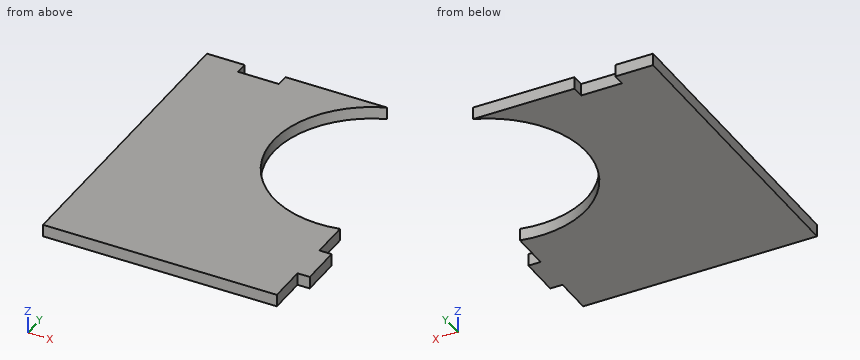
from build123d import *

# Parameters (mm, degrees)
SALIENTE_EXTRUIR1_DEPTH = 3


with BuildPart() as part:
    # Croquis1 → Saliente-Extruir1 (new body)
    with BuildSketch(Plane.XY):
        with BuildLine():
            Line((-3, 0.83840696), (-60.3, 0.83840696))
            Line((-60.3, 0.83840696), (-60.3, 75.83840696))
            Line((-60.3, 75.83840696), (-51.05, 75.83840696))
            Line((-51.05, 75.83840696), (-51.05, 72.83840696))
            Line((-51.05, 72.83840696), (-41.05, 72.83840696))
            Line((-41.05, 72.83840696), (-41.05, 75.83840696))
            Line((-41.05, 75.83840696), (-16.187910348, 75.83840696))
            ThreePointArc((-16.187910348, 75.83840696), (-30.919705343, 46.687711053), (-3, 29.73840696))
            Line((-3, 29.73840696), (-3, 20.28840696))
            Line((-3, 20.28840696), (0, 20.28840696))
            Line((0, 20.28840696), (0, 10.28840696))
            Line((0, 10.28840696), (-3, 10.28840696))
            Line((-3, 10.28840696), (-3, 0.83840696))
        make_face()
    extrude(amount=SALIENTE_EXTRUIR1_DEPTH)


solid = part.part
CAD build for the part. Positions are in the model's coordinates, mm. Give positions to 0.01 mm unless a question says otherwise; leave off trailing zeros. Loops run counter-clockwise (first coordinate to the right, second up) from the corner with the lowest first, then second, coordinate; pieces in that order, holes last. Notation, with made-up numbers: M 4.25,12.25 L 15.25,12.25 A32 cw 15.25,47.25 Z; hole C -27,-2 d5. An arc over 180 degrees is marked long. Write each question's results on one line, items separated by ' | '.
Q1. Band-saw the part on D-D on y = 32. Write the cut outline in (x, z), and give its area (3 significant figures).
Geometry check:
outline: M -60.3,0 L -18.96,0 L -18.96,3 L -60.3,3 Z | area: 124 mm²
Q2. Flat gauge pins, fed straight in: P1, Ø1.5, axis at y = 24.5, z = 1, coming from the +X side; P2, Ø1.5, axis at x = -1, z = 2, coming from the -Y side; P3, Ø1.5, axis at x = -2, z = 2, coming from the +Y side. Where does each tip first touch, or does it go through?
Geometry check:
P1: stops at x = -3 | P2: stops at y = 10.29 | P3: stops at y = 20.29
Q3. Band-saw the part on B-B on x = -25.5. Write the cut outline in (y, z).
Geometry check:
outline: M 0.84,0 L 37.02,0 L 37.02,3 L 0.84,3 Z; M 69.58,0 L 75.84,0 L 75.84,3 L 69.58,3 Z
Q4. Band-saw the part on C-C on x = -48. Write the cut outline in (y, z).
Geometry check:
outline: M 0.84,0 L 72.84,0 L 72.84,3 L 0.84,3 Z
Q5. Probe probe 1 along X at (y, z) = (24, 2.5); probe 2 along Y at (x, z) = (-21, 1); probe 3 along Y at (x, z) = (-45.5, 1.75). List the from-to ranges inside material, lowest first.
Geometry check:
probe 1: x = -60.3 to -3 | probe 2: y = 0.84 to 33.2, 73.4 to 75.84 | probe 3: y = 0.84 to 72.84
Q6. Band-saw the part on A-A on z = 1.35. Write the cut outline in (x, y).
Geometry check:
outline: M -60.3,0.84 L -3,0.84 L -3,10.29 L 0,10.29 L 0,20.29 L -3,20.29 L -3,29.74 A24.05 cw -16.19,75.84 L -41.05,75.84 L -41.05,72.84 L -51.05,72.84 L -51.05,75.84 L -60.3,75.84 Z
